Autodesk Inventor part; units mm, degrees
ref_plane "YZ Plane" through (0, 0, 0) normal (1, 0, 0) x (0, 1, 0)
ref_plane "XZ Plane" through (0, 0, 0) normal (0, 1, 0) x (-1, 0, 0)
ref_plane "XY Plane" through (0, 0, 0) normal (0, 0, 1) x (1, 0, 0)
sketch "Esquisse1" plane through (0, 0, 0) normal (0, 1, 0) x (-1, 0, 0)
  line L0 (-26.924, -14.7955) -> (26.924, -14.7955)
  line L1 (26.924, -14.7955) -> (26.924, 14.7955)
  line L2 (26.924, 14.7955) -> (-26.924, 14.7955)
  line L3 (-26.924, 14.7955) -> (-26.924, -14.7955)
  point P0 (0, 0)
  dimension "d0" = 29.591
  dimension "d1" = 53.848
  dimension "d2" = 26.924
  dimension "d3" = 14.7955
extrude "Extrusion1" add sketch "Esquisse1" along normal blind 20.32
fillet "Congé1" radius 2.54 4 edges at (-26.924, 10.16, 14.7955) (26.924, 10.16, 14.7955) (26.924, 10.16, -14.7955) (-26.924, 10.16, -14.7955)
shell "Coque1" thickness 1.5875 removed faces 1 at (-8.128, 20.32, -4.9318)
sketch "Esquisse3" plane through (0, 20.32, 0) normal (0, 1, 0) x (1, 0, 0)
  line L0 (-26.924, 12.2555) -> (-26.924, -12.2555)
  line L1 (-24.384, -14.7955) -> (24.384, -14.7955)
  line L2 (-15.8115, 11.1125) -> (12.7635, 11.1125)
  line L3 (12.7635, 11.1125) -> (12.7635, 17.4625)
  line L4 (12.7635, 17.4625) -> (-15.8115, 17.4625)
  line L5 (-15.8115, 17.4625) -> (-15.8115, 11.1125)
  line L6 (-15.8115, -11.1125) -> (12.7635, -11.1125)
  line L7 (12.7635, -11.1125) -> (12.7635, -17.4625)
  line L8 (12.7635, -17.4625) -> (-15.8115, -17.4625)
  line L9 (-15.8115, -17.4625) -> (-15.8115, -11.1125)
  point P0 (0, 0)
  dimension "d8" = 28.575
  dimension "d9" = 28.575
  dimension "d10" = 11.1125
  dimension "d11" = 11.1125
  dimension "d12" = 6.35
  dimension "d13" = 6.35
  dimension "d14" = 22.225
  dimension "d15" = 2.667
extrude "Extrusion2" cut sketch "Esquisse3" against normal blind 18.7325
sketch "Esquisse4" plane through (0, 20.32, 0) normal (0, 1, 0) x (1, 0, 0)
  line L0 (24.8732, 15.6385) -> (27.4132, 15.6385)
  line L1 (27.4132, 15.6385) -> (27.4132, -16.1115)
  line L2 (27.4132, -16.1115) -> (24.8732, -16.1115)
  line L3 (24.8732, -16.1115) -> (24.8732, 15.6385)
  point P0 (0, 0)
  dimension "d18" = 31.75
  dimension "d19" = 2.54
extrude "Extrusion3" cut sketch "Esquisse4" against normal blind 12.7
sketch "Esquisse5" plane through (25.3365, 1.5875, 12.2555) normal (0, 1, 0) x (1, 0, 0)
  line L0 (-50.673, 24.511) -> (-50.673, 0)
  line L1 (-12.573, -2.54) -> (-41.148, -2.54)
  circle A0 centre (-37.0205, 24.1808) radius 1.651
  circle A1 centre (-14.7955, 24.1808) radius 1.651
  circle A2 centre (-14.7955, 0.3556) radius 1.651
  circle A3 centre (-37.0205, 0.3556) radius 1.651
  circle A4 centre (-25.3365, 12.2555) radius 1.6
  line L2 (-49.7205, -2.54) -> (-41.148, -2.54)
  dimension "d22" = 3.302
  dimension "d23" = 3.302
  dimension "d24" = 3.302
  dimension "d25" = 3.302
  dimension "d26" = 3.2
  dimension "d27" = 23.8252
  dimension "d28" = 23.8252
  dimension "d29" = 22.225
  dimension "d30" = 22.225
  dimension "d31" = 2.8956
  dimension "d32" = 13.6525
  dimension "d33" = 2.8956
  dimension "d34" = 13.6525
extrude "Extrusion4" cut sketch "Esquisse5" against normal through all
equation "\"d9\" = d8"
equation "\"d11\" = d10"
equation "\"d23\" = d22"
equation "\"d24\" = d22"
equation "\"d25\" = d22"
equation "\"d28\" = d27"
equation "\"d30\" = d29"
equation "\"d33\" = d31"
equation "\"d34\" = d32"
properties part number "Batterie" material "Plastique ABS"
Check sheet for the modelled part. Datum: model origin and axes. Units: mm. A direction names the side the tool comes from. Round coordinates to 2 decimals unless told otherwise and drop trailing zeros. Order: outer loops, then holes, each group sorted by start corner. A loop starts at its lowest first (then second) coordinate and runs counter-clockwise, first axis right, second up. Notation, with made-up numbers: (-8, 3) - (39, 3) arc R9 cw to (39, 20) - close; hole circle Ø7 at (-10, 1.25). An arc over 180 degrees is marked (long way). Answer as CSV lines item,"result". Start each with the question number.
1) Tool access check on faces 1 (the face through (24.873, 14, -14)), 2 (the face through (11.43, 0.8, 10.51)), 3 (the face through (-20, 11, 13.208)). Record the directions out of +Z, -Z, +X, -X, +Y, -Y that give a thin tool (end or side, any length) a straight path to the whole face; none if there is none.
2) Section check B-B (y = 17.5). Record the cut outline in (x, z) (1 decimal), then the cut area to 3 significant figures.
3) Section check A-A (z = 0). Record the cut outline in (x, y), then the cut area to 3 significant figures.
4) Section check D-D (z = 8). Record the cut outline in (x, y).
5) Scan lines: probe 1 along X at (y, z) = (2.5, 9.5); probe 2 along Z at (x, y) = (0, 0.8); probe 3 along X at (y, z) = (0.6, 0). Record each from-to range of solid material in increasing order.
6) Depth check by flat-ended pin: pin 1 (1 mm diameter, centred on x = 25.5, z = -3.5, fed in from +Y); pin 2 (2.5 mm diameter, centred on x = -11.68, z = 11.9, fed in from +Y); pin 3 (1 mm diameter, centred on y = 14, z = 10.5, fed in from +X); pin 4 (1.3 mm diameter, centred on y = 9.5, z = 14, fed in from -X). Enter the tip coordinate at first touch or a pass-through.
7) Section check C-C (x = 0). Record the cut outline in (y, z), then the cut area to 3 significant figures.
8) Draft check along Z on faces 4 (the face through (-13.333, 0.805, -11.998)), 5 (the face through (-26.2, 10.3, 14.03)), 6 (the face through (25.336, 5, 0)), 7 (the face through (-26.924, 10, 0)). Enter one of: +Z half, -Z half, draft (parallel to the pull), parting line (faces both ways), or undercut.
Determined:
1,face 1,"+Z, -Z, +X, +Y"
1,face 2,"+Y, -Y"
1,face 3,"+Y"
2,outline,"(-26.9, -12.3) arc R2.5 ccw to (-24.4, -14.8) - (-15.8, -14.8) - (-15.8, -13.2) - (-24.4, -13.2) arc R1 cw to (-25.3, -12.3) - (-25.3, 12.3) arc R1 cw to (-24.4, 13.2) - (-15.8, 13.2) - (-15.8, 14.8) - (-24.4, 14.8) arc R2.5 ccw to (-26.9, 12.3) - close; (12.8, -14.8) - (24.4, -14.8) arc R2.5 ccw to (24.9, -14.7) - (24.9, -13.1) arc R1 cw to (24.4, -13.2) - (12.8, -13.2) - close; (12.8, 13.2) - (24.4, 13.2) arc R1 cw to (24.9, 13.1) - (24.9, 14.7) arc R2.5 ccw to (24.4, 14.8) - (12.8, 14.8) - close"
2,area,"113 mm^2"
3,outline,"(-26.92, 0) - (-1.6, 0) - (-1.6, 1.59) - (-25.34, 1.59) - (-25.34, 20.32) - (-26.92, 20.32) - close; (1.6, 0) - (26.92, 0) - (26.92, 7.62) - (25.34, 7.62) - (25.34, 1.59) - (1.6, 1.59) - close"
3,area,"120 mm^2"
4,outline,"(-26.92, 0) - (26.92, 0) - (26.92, 7.62) - (25.34, 7.62) - (25.34, 1.59) - (-25.34, 1.59) - (-25.34, 20.32) - (-26.92, 20.32) - close"
5,probe 1,"-26.92 to -25.34, 25.34 to 26.92"
5,probe 2,"-14.8 to -1.6, 1.6 to 14.8"
5,probe 3,"-26.92 to -1.6, 1.6 to 26.92"
6,pin 1,"y = 7.62"
6,pin 2,"through"
6,pin 3,"x = -25.34"
6,pin 4,"x = -26.68"
7,outline,"(0, -14.8) - (1.59, -14.8) - (1.59, -1.6) - (0, -1.6) - close; (0, 1.6) - (1.59, 1.6) - (1.59, 14.8) - (0, 14.8) - close"
7,area,"41.9 mm^2"
8,face 4,"undercut"
8,face 5,"+Z half"
8,face 6,"undercut"
8,face 7,"draft"
